The model under review builds one solid part; all positions refer to its coordinate system, in mm. A direction names the side the tool comes from. Coordinates: 2 decimals unless noted, no trailing zeros. Order: outer loops, then holes, each group sorted by start corner. A loop starts at its lowest first (then second) coordinate and runs counter-clockwise, first axis right, second up. Notation, with made-up numbers: (-8, -39.75) - (19, -39.75) arc R24 ccw to (19, -27.75) - close; hole circle Ø5 at (56.25, 23). An arc over 180 degrees is marked (long way). Answer in a Markdown table with one row per item.
```python
from build123d import *

# Parameters (mm, degrees)
F0_R     = 31.75
F0_R_2   = 3.175
F1_DEPTH = 31.75
F0_R_3   = 44.45
F2_DEPTH = 63.5
F3_SIZE2 = 28.575
F3_SIZE  = 2.54
F4_SIZE2 = 28.575
F4_SIZE  = 2.54


with BuildPart() as f1:
    # F0 (on Top) → F1 (new body)
    with BuildSketch(Plane.XY):
        Circle(F0_R)
        with BuildLine():
            ThreePointArc((3.175, -22.225), (-2.2450640303, -24.4700640303), (0, -19.05))
            ThreePointArc((0, -19.05), (2.2450640303, -19.9799359697), (3.175, -22.225))
        make_face(mode=Mode.SUBTRACT)
        with Locations((-22.225, 0)):
            Circle(F0_R_2, mode=Mode.SUBTRACT)
        with BuildLine():
            ThreePointArc((0, 13.9065), (9.8333804526, 9.8333804526), (13.9065, 0))
            ThreePointArc((13.9065, 0), (9.8333804526, -9.8333804526), (0, -13.9065))
            ThreePointArc((0, -13.9065), (-9.8333804526, -9.8333804526), (-13.9065, 0))
            ThreePointArc((-13.9065, 0), (-9.8333804526, 9.8333804526), (0, 13.9065))
        make_face(mode=Mode.SUBTRACT)
        with BuildLine():
            ThreePointArc((25.4, 0), (22.225, -3.175), (19.05, 0))
            ThreePointArc((19.05, 0), (22.225, 3.175), (25.4, 0))
        make_face(mode=Mode.SUBTRACT)
        with BuildLine():
            ThreePointArc((3.175, 22.225), (2.2450640303, 19.9799359697), (0, 19.05))
            ThreePointArc((0, 19.05), (-2.2450640303, 24.4700640303), (3.175, 22.225))
        make_face(mode=Mode.SUBTRACT)
    extrude(amount=F1_DEPTH)

    # F0 (on Top) → F2 (join)
    with BuildSketch(Plane.XY):
        Circle(F0_R_3)
        Circle(F0_R, mode=Mode.SUBTRACT)
    extrude(amount=F2_DEPTH)

    # F3
    f3_edges = [f1.edges().sort_by_distance(p)[0] for p in [
        (-44.45, 0, 63.5),
    ]]
    f3_side = f1.faces().sort_by_distance((-43.192764, 0, 63.5))[0]
    chamfer(f3_edges, length=F3_SIZE, length2=F3_SIZE2, reference=f3_side)

    # F4
    f4_edges = [f1.edges().sort_by_distance(p)[0] for p in [
        (0, -25.4, 0),
        (-25.4, 0, 0),
        (-13.9065, 0, 0),
        (19.05, 0, 0),
        (-3.175, 22.225, 0),
        (-44.45, 0, 0),
    ]]
    f4_side = f1.faces().sort_by_distance((0, -26.657236, 0))[0]
    chamfer(f4_edges, length=F4_SIZE, length2=F4_SIZE2, reference=f4_side)


solid = f1.part
```
Item 1: Clearance check with flat-ended pins moving along their axes: pin 1 Ø12 at (y, z) = (-32, 22.5) entering from +X; pin 2 Ø7.5 at (x, y) = (0, -22.225) entering from +Z; pin 3 Ø10 at (x, z) = (-34, 42) entering from +Y; pin 4 Ø10 at (x, y) = (6.5, -33) entering from -Z. State where each tip first meets the part, or that it passes through.
Check values:
| item | result |
|---|---|
| pin 1 | x = 35.43 |
| pin 2 | z = 31.75 |
| pin 3 | y = 32.89 |
| pin 4 | z = 0 |
Item 2: To check wall thickness, follow line 1 (X direction, y = 1, z = 31); line 2 (X direction, y = 2, z = 30); line 3 (Y direction, x = -19, z = 16). State the ranges of each line that lie inside material, in increasing order. Write a range as from..to.
Check values:
| item | result |
|---|---|
| line 1 | -44.44..-25.24, -19.21..-13.87, 13.87..19.21, 25.24..44.44 |
| line 2 | -44.4..-24.69, -19.76..-13.76, 13.76..19.76, 24.69..44.4 |
| line 3 | -38.94..-2.83, 2.83..38.94 |
Item 3: We need section A-A, the plane z = 21. Write out the cut boundary in (x, y) (3 decimals), then the cut area to 3 significant figures.
Check values:
| item | result |
|---|---|
| outline | circle Ø87.553 at (0, 0); hole circle Ø7.697 at (-22.225, 0); hole circle Ø29.16 at (0, 0); hole circle Ø7.697 at (0, -22.225); hole circle Ø7.697 at (0, 22.225); hole circle Ø7.697 at (22.225, 0) |
| area | 5,170 mm^2 |
Item 4: We need section B-B, the plane x = -2. State how many separate pieces and enclosed holes the cut face has, then the cut area to 3 significant figures.
Check values:
| item | result |
|---|---|
| separate pieces | 4 |
| enclosed holes | 0 |
| area | 2,050 mm^2 |
Item 5: We need section C-C, the plane z = 56.5. Write out the cut boundary in (x, y), then the cut area to 3 significant figures.
Check values:
| item | result |
|---|---|
| outline | circle Ø85.06 at (0, 0); hole circle Ø63.5 at (0, 0) |
| area | 2,520 mm^2 |
Item 6: Mouldability with a two-part tool opening along Y and no side actions: class faces 1 (the face through (-34.06, -26.11, 52.19)), 2 (the face through (9, -18, 0)), 3 (the face through (18.135, -1.696, 14.488)) as +Y half, -Y half, draft (parallel to the pull), parting line (faces both ways), or undercut.
Check values:
| item | result |
|---|---|
| face 1 | parting line |
| face 2 | draft |
| face 3 | undercut |
Item 7: Tool access review of faces 4 (the face through (14, -7, 31.75)), 5 (the face through (-34.06, -26.11, 11.31)): name each direction out of +Z, -Z, +X, -X, +Y, -Y from which nothing blocks a thin tool from reaching the whole face with its end or side.
Check values:
| item | result |
|---|---|
| face 4 | +Z |
| face 5 | -Z |
